Here's how the part is built. I have some questions about the finished solid (model axes, mm). A direction names the side the tool comes from. Coordinates: 2 decimals unless noted, no trailing zeros. Write each loop counter-clockwise with the first axis right and the second up, starting at its lowest first coordinate (ties: lowest second). Pieces come first, ordered by that corner, then holes.
Item 1: If we section it at A-A (y = 10): Please give me the cut outline in (x, z).
Item 2: We'd pull the mould along Z, two halves only. Please class faces 4 (the face through (-16.223, 22, -31)), 5 (the face through (20.795, 23.488, 21.183)), 6 (the face through (24.59, 2.46, -25.05)), 7 (the face through (24.59, 24.72, 25.05)): +Z half, -Z half, draft (parallel to the pull), parting line (faces both ways), or undercut.
Item 3: For faces 1 (the face through (24.59, 24.72, -25.05)), 2 (the face through (-14.472, 44.287, -25.785)), 3 (the face through (31.42, 2.465, 15.645)), which set-ups out of +Z, -Z, +X, -X, +Y, -Y let a thin tool reach every point of the face, with its end or its side?
Item 4: I'm going to push flat-ended pins straight in: pin 1 Ø11.5 at (y, z) = (28.5, 25) entering from -X; pin 2 Ø7 at (x, z) = (0.5, -2) entering from +Y; pin 3 Ø11 at (x, z) = (26, -2.5) entering from +Y; pin 4 Ø4 at (y, z) = (7, -37) entering from +X. Where does each tip first touch, or does it pass through?
Item 5: If I drill on line 1 (Y direction, x = 15.5, z = 9.5); line 2 (Z direction, x = 34.5, y = 21.5); line 3 (Z direction, x = 0, y = 1.6), over which ranges is the centre line in solid material (lowest first)?
Autodesk Inventor part; units mm, degrees
ref_plane "YZ Plane" through (0, 0, 0) normal (1, 0, 0) x (0, 1, 0)
ref_plane "XZ Plane" through (0, 0, 0) normal (0, 1, 0) x (-1, 0, 0)
ref_plane "XY Plane" through (0, 0, 0) normal (0, 0, 1) x (1, 0, 0)
sketch "Sketch1" plane through (0, 0, 0) normal (0, 1, 0) x (-1, 0, 0)
  circle A0 centre (0, 0) radius 52.5
  line L0 (52.5, 0) -> (16.2234, -49.9305)
  line L1 (16.2234, -49.9305) -> (-42.4734, -30.8587)
  line L2 (-42.4734, -30.8587) -> (-42.4734, 30.8587)
  line L3 (-42.4734, 30.8587) -> (16.2234, 49.9305)
  line L4 (16.2234, 49.9305) -> (52.5, 0)
  line L5 (52.5, 0) -> (-42.4734, 30.8587)
  line L6 (-42.4734, -30.8587) -> (52.5, 0)
  line L7 (16.2234, -49.9305) -> (16.2234, 49.9305)
  line L8 (-42.4734, -30.8587) -> (16.2234, 49.9305)
  line L9 (-42.4734, 30.8587) -> (16.2234, -49.9305)
  point P0 (16.2234, -11.787)
  point P1 (16.2234, 11.787)
  point P2 (-6.1968, 19.0717)
  point P3 (-20.0532, 0)
  point P4 (-6.1968, -19.0717)
extrude "Extrusion1" add sketch "Sketch1" along normal blind 5 contours L6 L7 L5 | L7 L5 L8 | L9 L6 L7 | L7 L6 L9 L8 L5 | L5 L8 L9 | L8 L9 L6
sketch "Sketch2" plane through (0, 5, 0) normal (0, 1, 0) x (1, 0, 0)
  circle A0 centre (0, 0) radius 4.25
  dimension "d3" = 8.5
extrude "Extrusion2" cut sketch "Sketch2" against normal blind 2
sketch "Sketch3" plane through (0, 3, 0) normal (0, 1, 0) x (1, 0, 0)
  circle A0 centre (0, 0) radius 2.5
  dimension "d6" = 5
extrude "Extrusion3" cut sketch "Sketch3" against normal through all
sketch "Sketch4" plane through (0, 5, 0) normal (0, 1, 0) x (1, 0, 0)
  line L0 (-16.2234, 11.787) -> (-52.5, 0)
  line L1 (-52.5, 0) -> (-16.2234, 11.787)
  line L2 (6.1968, 19.0717) -> (-16.2234, 49.9305)
  line L3 (-16.2234, 11.787) -> (-16.2234, 49.9305)
  line L4 (-16.2234, 49.9305) -> (6.1968, 19.0717)
  line L5 (42.4734, 30.8587) -> (6.1968, 19.0717)
  line L6 (6.1968, 19.0717) -> (42.4734, 30.8587)
  line L7 (42.4734, 30.8587) -> (20.0532, 0)
  line L8 (20.0532, 0) -> (42.4734, -30.8587)
  line L9 (-16.2234, -49.9305) -> (6.1968, -19.0717)
  line L10 (42.4734, -30.8587) -> (6.1968, -19.0717)
  line L11 (6.1968, -19.0717) -> (-16.2234, -49.9305)
  line L12 (-16.2234, -11.787) -> (-16.2234, -49.9305)
  line L13 (-16.2234, -49.9305) -> (-16.2234, -11.787)
  line L14 (-16.2234, -11.787) -> (-52.5, 0)
  line L15 (-52.5, 0) -> (-16.2234, -11.787)
  line L16 (-16.2234, -49.9305) -> (-15.4508, -47.5528)
  line L17 (-52.5, 0) -> (-44.4, 0)
  line L18 (-44.4, 0) -> (-13.7204, 42.2269)
  line L19 (-13.7204, 42.2269) -> (35.9204, 26.0977)
  line L20 (35.9204, 26.0977) -> (35.9204, -26.0977)
  line L21 (35.9204, -26.0977) -> (-13.7204, -42.2269)
  line L22 (-13.7204, -42.2269) -> (-44.4, 0)
  line L23 (-44.4, 0) -> (-13.7204, -42.2269)
  line L24 (-13.7204, -42.2269) -> (-13.7204, 42.2269)
  line L25 (-16.2234, -11.787) -> (-16.2234, -49.9305)
  line L26 (-13.7204, 42.2269) -> (35.9204, -26.0977)
  line L27 (35.9204, -26.0977) -> (-44.4, 0)
  line L28 (-44.4, 0) -> (35.9204, 26.0977)
  line L29 (35.9204, 26.0977) -> (-13.7204, -42.2269)
  line L30 (-16.2234, -49.9305) -> (6.1968, -19.0717)
  point P0 (0, 0)
  point P1 (0, 0)
  point P2 (5.2407, 16.1292)
  point P3 (16.9593, 0)
  point P4 (5.2407, -16.1292)
  point P5 (-13.7204, -9.9684)
  point P6 (-13.7204, 9.9684)
  dimension "d10" = 2.5
  dimension "d11" = 8.1
extrude "Extrusion4" add sketch "Sketch4" along normal blind 40 contours L3 L18 L24 L28 L0 | L18 L17 L0 | L3 L2 L19 L18 | L17 L22 L14 | L27 L24 L22 L12 L14 | L19 L2 L5 L28 L26 | L22 L21 L9 L12 | L29 L27 L21 L10 L9 | L5 L7 L20 L19 | L29 L20 L7 L8 L26 | L20 L8 L10 L21
fillet "Fillet1" radius 2.5 10 edges at (-13.7204, 45, 26.0977) (-29.0602, 45, 4.9842) (-29.0602, 45, -4.9842) (-13.7204, 45, -26.0977) (-4.2398, 45, -29.1781) (20.5805, 45, -21.1135) (26.4398, 45, -13.0488) (26.4398, 45, 13.0488) (20.5805, 45, 21.1135) (-4.2398, 45, 29.1781)
properties part number "StarP"
Answer list:
1. outline: (-52.5, 0) - (-16.22, -11.79) - (-16.22, -49.93) - (6.2, -19.07) - (42.47, -30.86) - (20.05, 0) - (42.47, 30.86) - (6.2, 19.07) - (-16.22, 49.93) - (-16.22, 11.79) - close; hole (-44.4, 0) - (-13.72, -9.97) - (-13.72, -42.23) - (5.24, -16.13) - (35.92, -26.1) - (16.96, 0) - (35.92, 26.1) - (5.24, 16.13) - (-13.72, 42.23) - (-13.72, 9.97) - close
2. face 4: draft
2. face 5: undercut
2. face 6: -Z half
2. face 7: +Z half
3. face 1: -Z, +Y, -Y
3. face 2: +Y
3. face 3: +X, +Y, -Y
4. pin 1: stops at x = -16.22
4. pin 2: stops at y = 5
4. pin 3: stops at y = 45
4. pin 4: stops at x = -5.38
5. line 1: y = 0 to 5
5. line 2: z = -28.27 to -25.64, -24.14 to -19.88, 19.88 to 24.14, 25.64 to 28.27
5. line 3: z = -27.6 to -2.5, 2.5 to 27.6
